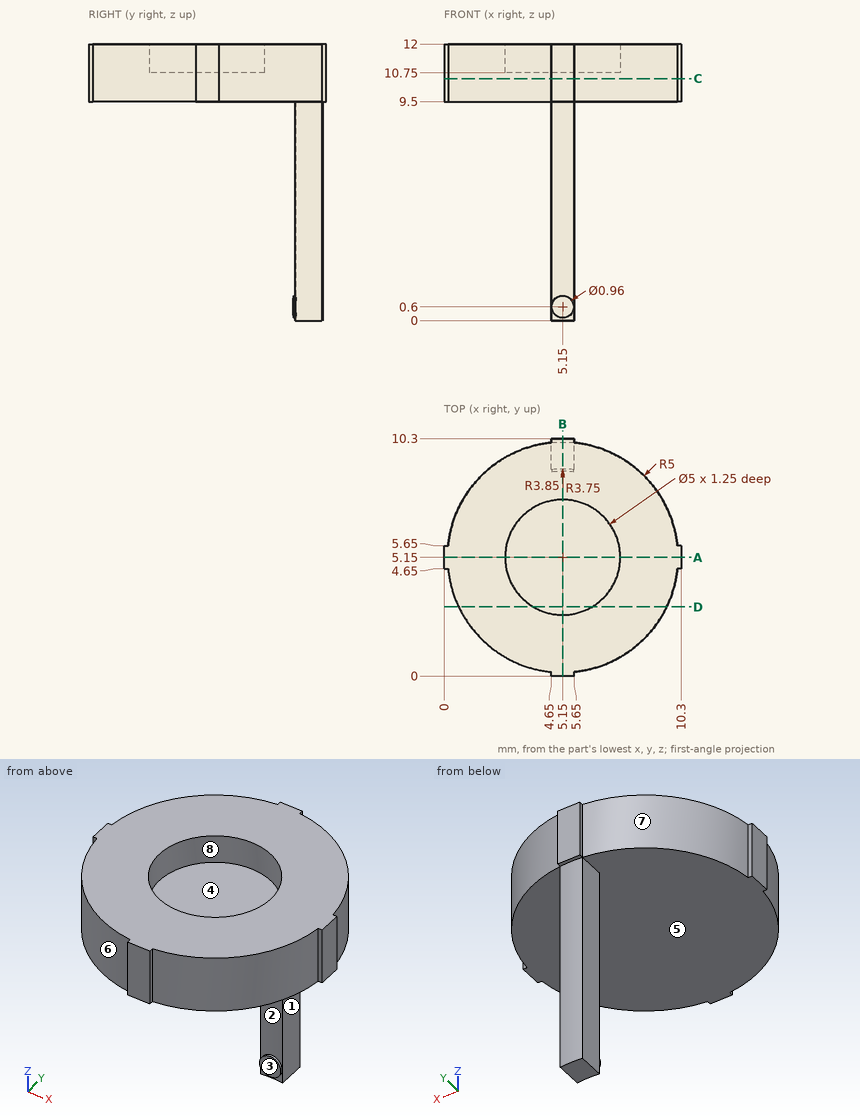
Geometry: see drawing. Coordinates: mm, zero at the bounding-box minimum. A direction names the side the tool comes from. Round coordinates to 2 decimals unless told otherwise and drop trailing zeros. Loops run counter-clockwise (first coordinate to the right, second up) from the corner with the lowest first, then second, coordinate; pieces in that order, holes last. Notation, with made-up numbers: (18, 25.25) - (54, 25.25) arc R21 ccw to (54, 45.25) - close; hole circle Ø5 at (46, 53). An arc over 180 degrees is marked (long way). One line per item, written item: value. Start each with the question number.
(1) Section A-A, the plane y = 5.15. Return loops of the section in (x, z).
(2) Ray query, line 1 (Y direction, x = 5.15, z = 11.7); line 2 (Z direction, x = 8, y = 4.5); line 3 (Z direction, x = 4.25, y = 3.75). Return the intervals inside material, ascending. Write a range as [from, to].
(3) Section C-C, the plane z = 10.5. Return loops of the section in (x, y).
(4) Section D-D, the plane y = 3. Return loops of the section in (x, z), plus the area to 3 significant figures.
(5) Section B-B, the plane x = 5.15. Return loops of the section in (y, z), plus the area to 3 significant figures.
(6) Contact query for flat-ended pins moving along their axis: P1, Ø3, axis at x = 7, z = 2, coming from the -Y side; P2, Ø0.6, axis at y = 9.5, z = 3, coming from the -X side; P3, Ø3, axis at x = 3, y = 4, coming from the -Z side. Output: stop coordinate, or through.
(7) Draft query along Y for the marked faces 5, 6, 7 and 8. Return one class per face: +Y half, -Y half, draft (parallel to the pull), parting line (faces both ways), or undercut.
(8) Access query for the marked faces 1, 2, 3 and 4. Directions: +Z, -Z, +X, -X, +Y, -Y. A direction counts if a zero-diameter tool reaches every point of the face in a straight line with its end or side. Return the directions, or none.
Results below:
1. outline: (0, 9.5) - (10.3, 9.5) - (10.3, 12) - (7.65, 12) - (7.65, 10.75) - (2.65, 10.75) - (2.65, 12) - (0, 12) - close
2. line 1: [0, 2.65], [7.65, 10.3]
2. line 2: [9.5, 12]
2. line 3: [9.5, 10.75]
3. outline: (0, 4.65) - (0.18, 4.65) arc R5 ccw to (4.65, 0.18) - (4.65, 0) - (5.65, 0) - (5.65, 0.18) arc R5 ccw to (10.12, 4.65) - (10.3, 4.65) - (10.3, 5.65) - (10.12, 5.65) arc R5 ccw to (5.65, 10.12) - (5.65, 10.3) - (4.65, 10.3) - (4.65, 10.12) arc R5 ccw to (0.18, 5.65) - (0, 5.65) - close
4. outline: (0.64, 9.5) - (9.66, 9.5) - (9.66, 12) - (6.43, 12) - (6.43, 10.75) - (3.87, 10.75) - (3.87, 12) - (0.64, 12) - close
4. area: 19.4 mm^2
5. outline: (0, 9.5) - (9, 9.5) - (9, 1.08) - (8.9, 1.08) - (8.9, 0.12) - (9, 0.12) - (9, 0) - (10.15, 0) - (10.15, 9.5) - (10.3, 9.5) - (10.3, 12) - (7.65, 12) - (7.65, 10.75) - (2.65, 10.75) - (2.65, 12) - (0, 12) - close
5. area: 30.5 mm^2
6. P1: y = 8.97
6. P2: x = 4.65
6. P3: z = 9.5
7. face 5: draft
7. face 6: -Y half
7. face 7: +Y half
7. face 8: undercut
8. face 1: -Z, +X, +Y, -Y
8. face 2: -Y
8. face 3: -Z, -Y
8. face 4: +Z
